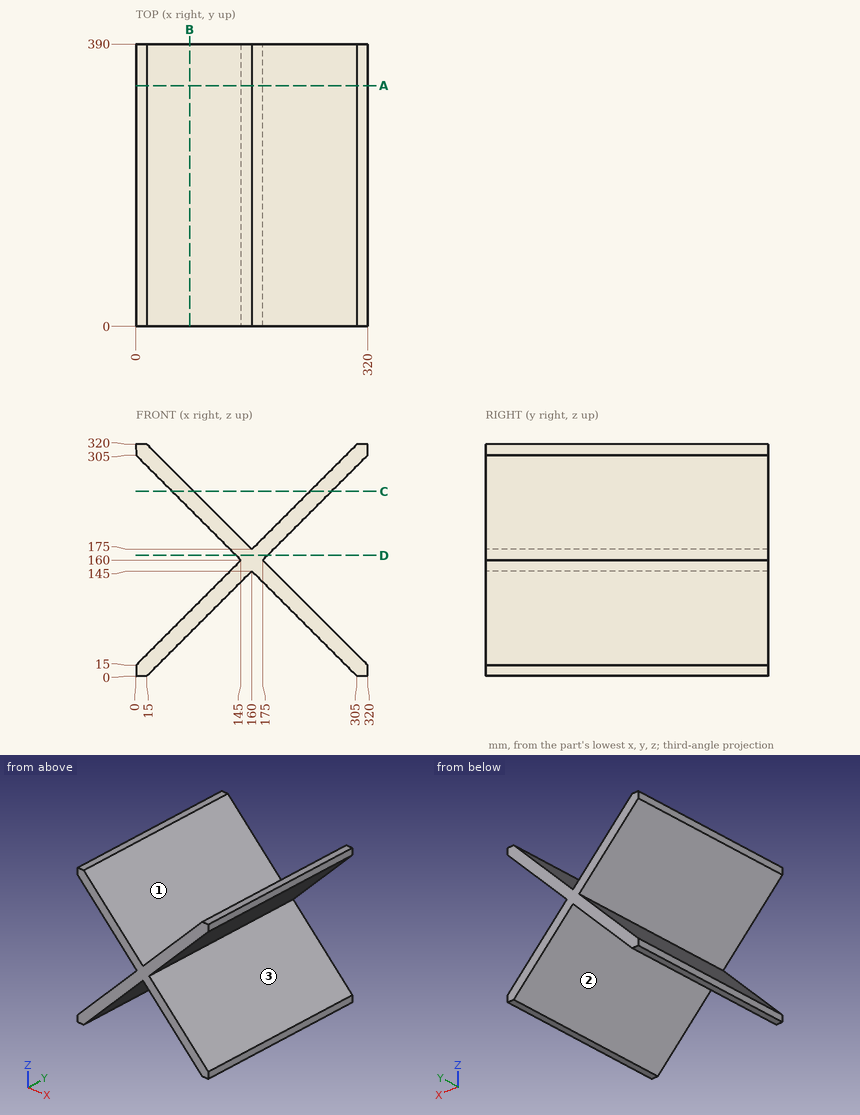
Answer from the drawing. Dimensions are ordinates in mm from the lowest x, y and z of the part. Coordinates: 2 decimals unless noted, no trailing zeros. Loops run counter-clockwise (first coordinate to the right, second up) from the corner with the lowest first, then second, coordinate; pieces in that order, holes last. Notation, with made-up numbers: (12, 31.25) - (49, 31.25) arc R18 ccw to (49, 38.25) - close; hole circle Ø2 at (34, 5). An arc over 180 degrees is marked (long way). Use a Markdown table: item, result.
Item 1: Find section A-A, the plane y = 332.5. Determine the outline of the cut face in (x, z).
Evaluation:
| item | result |
|---|---|
| outline | (0, 0) - (15, 0) - (160, 145) - (305, 0) - (320, 0) - (320, 15) - (175, 160) - (320, 305) - (320, 320) - (305, 320) - (160, 175) - (15, 320) - (0, 320) - (0, 305) - (145, 160) - (0, 15) - close |
Item 2: Find section B-B, the plane x = 74. Determine the outline of the cut face in (y, z), and give its area (3 significant figures).
Evaluation:
| item | result |
|---|---|
| outline | (0, 59) - (390, 59) - (390, 89) - (0, 89) - close; (0, 231) - (390, 231) - (390, 261) - (0, 261) - close |
| area | 23,400 mm2 |
Item 3: Find section D-D, the plane z = 166.5. Determine the outline of the cut face in (x, y), and give its area (3 significant figures).
Evaluation:
| item | result |
|---|---|
| outline | (138.5, 0) - (181.5, 0) - (181.5, 390) - (138.5, 390) - close |
| area | 16,800 mm2 |
Item 4: The mould has two halves that part along Z. Classify the marked faces 1, 2 and 3: +Z half, -Z half, draft (parallel to the pull), parting line (faces both ways), or undercut.
Evaluation:
| item | result |
|---|---|
| face 1 | +Z half |
| face 2 | -Z half |
| face 3 | undercut |
Item 5: Given pin 1 Ø1.5 at (y, z) = (327.5, 163) entering from -X; pin 2 Ø2 at (x, y) = (90, 88.5) entering from +Z; pin 3 Ø4 at (y, z) = (332.5, 220) entering from -X, each flat-ended and moving along its own axis, determine where each tip first touches the part or whether it passes through.
Evaluation:
| item | result |
|---|---|
| pin 1 | stops at x = 141.25 |
| pin 2 | stops at z = 246 |
| pin 3 | stops at x = 83 |
Item 6: Find section C-C, the plane z = 255. Determine the outline of the cut face in (x, y).
Evaluation:
| item | result |
|---|---|
| outline | (50, 0) - (80, 0) - (80, 390) - (50, 390) - close; (240, 0) - (270, 0) - (270, 390) - (240, 390) - close |
Item 7: Consider probe 1 along X at (y, z) = (283.5, 80); probe 2 along X at (y, z) = (357.5, 231); probe 3 along Z at (x, y) = (202, 166.5). Determine where each line is inside the solid, lowest interval first. Write a range as from..to.
Evaluation:
| item | result |
|---|---|
| probe 1 | x = 65..95, 225..255 |
| probe 2 | x = 74..104, 216..246 |
| probe 3 | z = 103..133, 187..217 |
